from build123d import *

# Parameters (mm, degrees)
BOSS_EXTRU_1_DEPTH = 0.1
ESQUISSE2_W        = 1.2
ESQUISSE2_H        = 1.2
BOSS_EXTRU_2_DEPTH = 0.1


with BuildPart() as part:
    # Esquisse1 → Boss.-Extru.1 (new body)
    with BuildSketch(Plane.XY):
        with BuildLine():
            Line((0, -0.5), (6.9, -0.5))
            ThreePointArc((6.9, -0.5), (7.253553391, -0.353553391), (7.4, 0))
            Line((7.4, 0), (7.4, 5.9))
            ThreePointArc((7.4, 5.9), (7.253553391, 6.253553391), (6.9, 6.4))
            Line((6.9, 6.4), (0, 6.4))
            ThreePointArc((0, 6.4), (-0.353553391, 6.253553391), (-0.5, 5.9))
            Line((-0.5, 5.9), (-0.5, 0))
            ThreePointArc((-0.5, 0), (-0.353553391, -0.353553391), (0, -0.5))
        make_face()
    extrude(amount=BOSS_EXTRU_1_DEPTH)

    # Esquisse2 → Boss.-Extru.2 (add)
    with BuildSketch(Plane.XY.offset(0.1)):
        with Locations((1.3, 0.7)):
            Rectangle(ESQUISSE2_W, ESQUISSE2_H)
        with Locations((2.733333333, 0.7)):
            Rectangle(ESQUISSE2_W, ESQUISSE2_H)
        with Locations((4.166666667, 0.7)):
            Rectangle(ESQUISSE2_W, ESQUISSE2_H)
        with Locations((5.6, 0.7)):
            Rectangle(ESQUISSE2_W, ESQUISSE2_H)
        with Locations((2.733333333, 2.2)):
            Rectangle(ESQUISSE2_W, ESQUISSE2_H)
        with Locations((4.166666667, 2.2)):
            Rectangle(ESQUISSE2_W, ESQUISSE2_H)
        with Locations((5.6, 2.2)):
            Rectangle(ESQUISSE2_W, ESQUISSE2_H)
        with Locations((2.733333333, 3.7)):
            Rectangle(ESQUISSE2_W, ESQUISSE2_H)
        with Locations((4.166666667, 3.7)):
            Rectangle(ESQUISSE2_W, ESQUISSE2_H)
        with Locations((5.6, 3.7)):
            Rectangle(ESQUISSE2_W, ESQUISSE2_H)
        with Locations((2.733333333, 5.2)):
            Rectangle(ESQUISSE2_W, ESQUISSE2_H)
        with Locations((4.166666667, 5.2)):
            Rectangle(ESQUISSE2_W, ESQUISSE2_H)
        with Locations((5.6, 5.2)):
            Rectangle(ESQUISSE2_W, ESQUISSE2_H)
        with Locations((1.3, 2.2)):
            Rectangle(ESQUISSE2_W, ESQUISSE2_H)
        with Locations((1.3, 3.7)):
            Rectangle(ESQUISSE2_W, ESQUISSE2_H)
        with Locations((1.3, 5.2)):
            Rectangle(ESQUISSE2_W, ESQUISSE2_H)
    extrude(amount=BOSS_EXTRU_2_DEPTH)


solid = part.part
Could you check a few things on this model? Use its own coordinates, in mm. Coordinates: 2 decimals unless noted, no trailing zeros. Loops run counter-clockwise (first coordinate to the right, second up) from the corner with the lowest first, then second, coordinate; pieces in that order, holes last.
1. For P1, Ø2, axis at x = 3, y = 1.5, coming from the -Z side, with a flat end and sliding along its axis, tell me the tip position at first contact or that it passes through.
2. Imagine slicing it at D-D (y = 3). Please give me the cut outline in (x, z).
3. Imagine slicing it at C-C (z = 0.15). Give the number of separate pieces and of enclosed holes in the cut face, and give its area (3 significant figures).
4. Imagine slicing it at A-A (y = 0.25). Please give me the cut outline in (x, z).
5. Imagine slicing it at B-B (x = 5.5). Please give me the cut outline in (y, z).
6. I need wall thicknesses on L1, parallel to X at y = 2, z = 0.15; L2, parallel to Y at x = 1.5, z = 0.15. Which ranges of each line are inside material? Lowest first, please.
Computed values:
1. P1: stops at z = 0
2. outline: (-0.5, 0) - (7.4, 0) - (7.4, 0.1) - (-0.5, 0.1) - close
3. separate pieces: 16
3. enclosed holes: 0
3. area: 23.0 mm2
4. outline: (-0.5, 0) - (7.4, 0) - (7.4, 0.1) - (6.2, 0.1) - (6.2, 0.2) - (5, 0.2) - (5, 0.1) - (4.77, 0.1) - (4.77, 0.2) - (3.57, 0.2) - (3.57, 0.1) - (3.33, 0.1) - (3.33, 0.2) - (2.13, 0.2) - (2.13, 0.1) - (1.9, 0.1) - (1.9, 0.2) - (0.7, 0.2) - (0.7, 0.1) - (-0.5, 0.1) - close
5. outline: (-0.5, 0) - (6.4, 0) - (6.4, 0.1) - (5.8, 0.1) - (5.8, 0.2) - (4.6, 0.2) - (4.6, 0.1) - (4.3, 0.1) - (4.3, 0.2) - (3.1, 0.2) - (3.1, 0.1) - (2.8, 0.1) - (2.8, 0.2) - (1.6, 0.2) - (1.6, 0.1) - (1.3, 0.1) - (1.3, 0.2) - (0.1, 0.2) - (0.1, 0.1) - (-0.5, 0.1) - close
6. L1: x = 0.7 to 1.9, 2.13 to 3.33, 3.57 to 4.77, 5 to 6.2
6. L2: y = 0.1 to 1.3, 1.6 to 2.8, 3.1 to 4.3, 4.6 to 5.8
